The model under review builds one solid part; all positions refer to its coordinate system, in mm. Coordinates: 2 decimals unless noted, no trailing zeros. Order: outer loops, then holes, each group sorted by start corner. A loop starts at its lowest first (then second) coordinate and runs counter-clockwise, first axis right, second up. Notation, with made-up numbers: (27, 47.5) -> (77, 47.5) arc R19 cw to (77, 71.5) -> close; hole circle Ø7 at (80, 72.5). An arc over 180 degrees is marked (long way). Put each result on its own line as item: value.
Solid Edge part; units mm, degrees
sketch "Sketch1" plane through (0, 0, 0) normal (0, -1, 0) x (1, 0, 0)
  line L0 (-42.5, 0) -> (42.5, 0)
  line L1 (42.5, 0) -> (42.5, 76)
  line L2 (42.5, 76) -> (-42.5, 76)
  line L3 (-42.5, 76) -> (-42.5, 0)
  circle A0 centre (28.5, 68) radius 3.3
  circle A1 centre (0, 68) radius 3.3
  circle A2 centre (-28.5, 68) radius 3.3
  circle A3 centre (28.5, 8) radius 3.3
  circle A4 centre (0, 8) radius 3.3
  circle A5 centre (-28.5, 8) radius 3.3
  dimension "D1" = 42.5
extrude "Protrusion1" add sketch "Sketch1" along normal blind 10
Item 1: Consider section B-B on y = -2.25. Write out the cut boundary in (x, z), and give its area (3 significant figures).
Answers below:
outline: (-42.5, 0) -> (42.5, 0) -> (42.5, 76) -> (-42.5, 76) -> close; hole circle Ø6.6 at (-28.5, 8); hole circle Ø6.6 at (-28.5, 68); hole circle Ø6.6 at (0, 8); hole circle Ø6.6 at (0, 68); hole circle Ø6.6 at (28.5, 8); hole circle Ø6.6 at (28.5, 68)
area: 6,250 mm^2
Item 2: Consider section A-A on z = 8. Write out the cut boundary in (x, y).
Answers below:
outline: (-42.5, -10) -> (-31.8, -10) -> (-31.8, 0) -> (-42.5, 0) -> close; (-25.2, -10) -> (-3.3, -10) -> (-3.3, 0) -> (-25.2, 0) -> close; (3.3, -10) -> (25.2, -10) -> (25.2, 0) -> (3.3, 0) -> close; (31.8, -10) -> (42.5, -10) -> (42.5, 0) -> (31.8, 0) -> close
Item 3: For pin 1 Ø6 at (x, z) = (-28.5, 68) entering from +Y, flat-tipped, find the tip position at first contact; note if it passes through.
Answers below:
pin 1: through
Item 4: For line 1 (Z direction, x = 28.5, y = -7); line 2 (X direction, y = -8, z = 66.5), list the stretches that pass through material, from the lowest coordinate up. Write a range as from..to.
Answers below:
line 1: 0..4.7, 11.3..64.7, 71.3..76
line 2: -42.5..-31.44, -25.56..-2.94, 2.94..25.56, 31.44..42.5
Item 5: Consider section C-C on x = -28.5. Write out the cut boundary in (y, z).
Answers below:
outline: (-10, 0) -> (0, 0) -> (0, 4.7) -> (-10, 4.7) -> close; (-10, 11.3) -> (0, 11.3) -> (0, 64.7) -> (-10, 64.7) -> close; (-10, 71.3) -> (0, 71.3) -> (0, 76) -> (-10, 76) -> close
Item 6: Mouldability with a two-part tool opening along Z and no side actions: class faces 1 (the cylindrical face through (-26.726, -4.93, 65.217)), 2 (the flat face through (-42.5, -5, 39)), 3 (the flat face through (-1, -5, 0)) as +Z half, -Z half, draft (parallel to the pull), parting line (faces both ways), or undercut.
Answers below:
face 1: undercut
face 2: draft
face 3: -Z half
